Design review of the part built by this model. Coordinates are the model's own, in mm. Coordinates: 2 decimals unless noted, no trailing zeros. Loops run counter-clockwise (first coordinate to the right, second up) from the corner with the lowest first, then second, coordinate; pieces in that order, holes last. Notation, with made-up numbers: (19.25, 48.5) - (74.25, 48.5) arc R22 cw to (74.25, 71.5) - close; hole circle Ø3 at (6.5, 82). An arc over 180 degrees is marked (long way). One line per question, with ' | ' between items.
Autodesk Inventor part; units mm, degrees
ref_plane "YZ Plane" through (0, 0, 0) normal (1, 0, 0) x (0, 1, 0)
ref_plane "XZ Plane" through (0, 0, 0) normal (0, 1, 0) x (-1, 0, 0)
ref_plane "XY Plane" through (0, 0, 0) normal (0, 0, 1) x (1, 0, 0)
sketch "Sketch1" plane through (0, 0, 0) normal (0, 0, 1) x (1, 0, 0)
  circle A0 centre (0, 0) radius 77.5
  circle A1 centre (0, 0) radius 40
  dimension "d22" = 155
  dimension "d23" = 80
extrude "Plate1" add sketch "Sketch1" along normal blind 6
sketch "Sketch5" plane through (0, 0, 6) normal (0, 0, 1) x (1, 0, 0)
  circle A0 centre (0, -62.5) radius 8.5
  point P0 (0, 0)
  dimension "d24" = 62.5
  dimension "d25" = 17
extrude "Cut1" cut sketch "Sketch5" against normal blind 6
pattern_circular "Circular Pattern1" count 4 over 360 about axis through (0, 0, 0) along (0, 0, 1) of "Cut1"
equation "\"d26\" = Thickness"
equation "\"d2\" = Thickness"
equation "\"BendReliefWidth\" = Thickness"
equation "\"BendReliefDepth\" = 0.5 * Thickness"
equation "\"CornerReliefSize\" = 4 * Thickness"
equation "\"MinimumRemnant\" = 2 * Thickness"
equation "\"TransitionRadius\" = BendRadius"
equation "\"JacobiRadiusSize\" = BendRadius"
equation "\"GapSize\" = Thickness"
properties part number "Flange DN 50" material "Steel"
Q1. Take a section at D-D (y = -60.5). Give the boundary of the cut face in (x, z).
Returned:
outline: (-48.44, 0) - (-8.26, 0) - (-8.26, 6) - (-48.44, 6) - close; (8.26, 0) - (48.44, 0) - (48.44, 6) - (8.26, 6) - close
Q2. Draft analysis for pull direction Y (two halves, no side actions). For faces 1 (the cylindrical face through (-8.67, 39.05, 2.96)), 2 (the cylindrical face through (-67.672, 6.745, 3.042)), 3 (the flat face through (33, -33, 6)), 4 (the cylindrical face through (-16.8, 75.657, 2.958)), state which applies: +Y half, -Y half, draft (parallel to the pull), parting line (faces both ways), or undercut.
Returned:
face 1: undercut | face 2: undercut | face 3: draft | face 4: parting line
Q3. Take a section at C-C (x = -22). Give the boundary of the cut face in (y, z).
Returned:
outline: (-74.31, 0) - (-33.41, 0) - (-33.41, 6) - (-74.31, 6) - close; (33.41, 0) - (74.31, 0) - (74.31, 6) - (33.41, 6) - close
Q4. To check wall thickness, follow line 1 along Y through (x, z) = (0, 3.25); line 2 along X through (y, z) = (-3.5, 5.2); line 3 along X through (y, z) = (27, 3.4). State the ranges of each line that lie inside material, in increasing order.
Returned:
line 1: y = -77.5 to -71, -54 to -40, 40 to 54, 71 to 77.5 | line 2: x = -77.42 to -70.25, -54.75 to -39.85, 39.85 to 54.75, 70.25 to 77.42 | line 3: x = -72.64 to -29.51, 29.51 to 72.64
Q5. For pin 1 (3 mm diameter, centred on y = -56, z = 4.5, fed in from +X); pin 2 (3 mm diameter, centred on y = -39.5, z = 2, fed in from -X), all flat-tipped, find the tip position at first contact; note any pin that passes through.
Returned:
pin 1: stops at x = 55.1 | pin 2: stops at x = -67.54
Q6. Take a section at A-A (y = 0). Give the boundary of the cut face in (x, z).
Returned:
outline: (-77.5, 0) - (-71, 0) - (-71, 6) - (-77.5, 6) - close; (-54, 0) - (-40, 0) - (-40, 6) - (-54, 6) - close; (40, 0) - (54, 0) - (54, 6) - (40, 6) - close; (71, 0) - (77.5, 0) - (77.5, 6) - (71, 6) - close
